Verification items for the finished model (mm, model axes). A direction names the side the tool comes from. Round coordinates to 2 decimals unless told otherwise and drop trailing zeros. Write each loop counter-clockwise with the first axis right and the second up, starting at its lowest first coordinate (ties: lowest second). Pieces come first, ordered by that corner, then holes. Notation, with made-up numbers: (-4, -19.5) - (21, -19.5) arc R19 cw to (21, -3.5) - close; hole circle Ø3 at (0.5, 52). An arc over 180 degrees is marked (long way). Answer as a JSON object with one key per item and string values. Group by question number.
1) Go/stop test with flat-tipped pins: pin 1 Ø2 at (y, z) = (239.5, 174.5) entering from +X; pin 2 Ø2 at (x, y) = (150, 169) entering from -Z. Record where each tip stops, or that it passes through.
2) Thickness scan on line 1 (Z direction, x = 230.5, y = 75); line 2 (X direction, y = 247.5, z = -128.5); line 3 (Z direction, x = -428, y = 171). Record the ranges inside material, lowest first.
3) Mould release check, pull along X, two halves, no side actions. Record for faces 3 (the flat face through (-60, 142, 219.562)), 4 (the cylindrical face through (-484.01, 269.28, 57.36)), 5 (the cylindrical face through (-310.902, 39.118, -134.088)): +X half, -X half, draft (parallel to the pull), parting line (faces both ways), or undercut.
4) Section check D-D (y = 215.5). Enter the section's corners in (x, z).
5) Set-up check for faces 1 (the cylindrical face through (-310.9, 260.37, -134.09)), 2 (the cylindrical face through (-484.014, 146.016, 200.841)): record each of +Z, -Z, +X, -X, +Y, -Y from which the full face is reachable in a straight line by a thin tool's end or side.
6) Section check B-B (x = -90). Enter the section's corners in (y, z).
7) Section check C-C (z = 181.5). Enter the section's corners in (x, y).
8) Section check A-A (y = 132). Enter the section's corners in (x, z), then the cut area to 3 significant figures.
```python
from build123d import *

# Parameters (mm, degrees)
F0_W     = 1044
F0_H     = 329
F1_DEPTH = 288
F2_R     = 100
F4_DEPTH = 288.001
F5_R     = 15
F6_DEPTH = 50


with BuildPart() as f1:
    # F0 (on Front) → F1 (new body)
    with BuildSketch(Plane.XZ):
        with Locations((-3.758688, 55.06163)):
            Rectangle(F0_W, F0_H)
    extrude(amount=-F1_DEPTH)

    # F2
    f2_edges = [f1.edges().sort_by_distance(p)[0] for p in [
        (-525.758688, 144, 219.56163),
        (-525.758688, 144, -109.43837),
        (-525.758688, 0, 55.06163),
        (-525.758688, 288, 55.06163),
    ]]
    fillet(f2_edges, radius=F2_R)

    # F3 (on face) → F4 (cut, through all)
    with BuildSketch(Plane.XZ):
        Polygon((518.241312, 219.56163), (317.040984, 219.56163), (518.241312, 125.740376), align=None)
    extrude(amount=-F4_DEPTH, mode=Mode.SUBTRACT)

    # F5 (on face) → F6 (join)
    with BuildSketch(Plane(origin=(0, 0, -109.43837), x_dir=(1, 0, 0), z_dir=(0, 0, -1))):
        with Locations((-324.758688, -33.373285)):
            Circle(F5_R)
        with Locations((146.241312, -31.188212)):
            Circle(F5_R)
        with Locations((-324.758688, -254.626715)):
            Circle(F5_R)
        with Locations((146.241312, -256.811788)):
            Circle(F5_R)
    extrude(amount=F6_DEPTH)


solid = f1.part
```
Returned:
{
 "1": {"pin 1": "x = 415.82", "pin 2": "z = -109.44"},
 "2": {"line 1": "-109.44 to 219.56", "line 2": "-337.96 to -311.56, 134.48 to 158", "line 3": "-109.41 to 219.54"},
 "3": {"face 3": "draft", "face 4": "-X half", "face 5": "undercut"},
 "4": {"outline": "(-521.9, -36.94) arc R100 ccw to (-425.76, -109.44) - (518.24, -109.44) - (518.24, 125.74) - (317.04, 219.56) - (-425.76, 219.56) arc R100 ccw to (-521.9, 147.06) - close"},
 "5": {"face 1": "-Z", "face 2": "+Z, -X, +Y, -Y"},
 "6": {"outline": "(0, -109.44) - (288, -109.44) - (288, 219.56) - (0, 219.56) - close"},
 "7": {"outline": "(-504.27, 38.06) arc R100 ccw to (-425.76, 0) - (398.66, 0) - (398.66, 288) - (-425.76, 288) arc R100 ccw to (-504.27, 249.94) - close"},
 "8": {"outline": "(-525.76, -9.44) arc R100 ccw to (-425.76, -109.44) - (518.24, -109.44) - (518.24, 125.74) - (317.04, 219.56) - (-425.76, 219.56) arc R100 ccw to (-525.76, 119.56) - close", "area": "330,000 mm2"}
}
